Read the model definition and answer for the solid it produces. Units are mm, in the model's axes. Coordinates: 2 decimals unless noted, no trailing zeros. Order: outer loops, then holes, each group sorted by start corner. A loop starts at its lowest first (then second) coordinate and runs counter-clockwise, first axis right, second up. Notation, with made-up numbers: (-23, 33) - (17, 33) arc R12 cw to (17, 37) - close; hole circle Ø4 at (83, -3). An arc over 180 degrees is marked (long way). Answer as a JSON object with one key per item and string values. Group by question number.
from build123d import *

# Parameters (mm, degrees)
BOSS_EXTRUDE1_DEPTH = 3
SKETCH2_R           = 1.95
CUT_EXTRUDE1_DEPTH  = 4


with BuildPart() as part:
    # Sketch1 → Boss-Extrude1 (new body)
    with BuildSketch(Plane(origin=(0, 0, 0), x_dir=(1, 0, 0), z_dir=(0, 1, 0))):
        with BuildLine():
            Line((-54, 0), (-2, 0))
            ThreePointArc((-2, 0), (-0.585786438, -0.585786438), (0, -2))
            Line((0, -2), (0, -13))
            ThreePointArc((0, -13), (-0.585786438, -14.414213562), (-2, -15))
            Line((-2, -15), (-54, -15))
            ThreePointArc((-54, -15), (-55.414213562, -14.414213562), (-56, -13))
            Line((-56, -13), (-56, -2))
            ThreePointArc((-56, -2), (-55.414213562, -0.585786438), (-54, 0))
        make_face()
    extrude(amount=BOSS_EXTRUDE1_DEPTH)

    # Sketch2 → Cut-Extrude1 (cut, through all)
    with BuildSketch(Plane(origin=(0, 3, 0), x_dir=(1, 0, 0), z_dir=(0, 1, 0))):
        with Locations((-4, -4)):
            Circle(SKETCH2_R)
        with Locations((-12, -4)):
            Circle(SKETCH2_R)
        with Locations((-76, -4)):
            Circle(SKETCH2_R)
        with Locations((-68, -4)):
            Circle(SKETCH2_R)
        with Locations((-60, -4)):
            Circle(SKETCH2_R)
        with Locations((-52, -4)):
            Circle(SKETCH2_R)
        with Locations((-44, -4)):
            Circle(SKETCH2_R)
        with Locations((-36, -4)):
            Circle(SKETCH2_R)
        with Locations((-28, -4)):
            Circle(SKETCH2_R)
        with Locations((-20, -4)):
            Circle(SKETCH2_R)
    extrude(amount=-CUT_EXTRUDE1_DEPTH, mode=Mode.SUBTRACT)


solid = part.part
1. A cutting plane is placed at B-B on y = 1.7. Write down the section's boundary in (x, z), and give its area (3 significant figures).
2. A cutting plane is placed at C-C on z = 4. State how many separate pieces and enclosed holes the cut face has, and give its area (3 significant figures).
3. Straight lines are drawn through the part: L1, parallel to Z at x = -52, y = 1.5; L2, parallel to Z at x = -29, y = 0.6; L3, parallel to X at y = 1.1, z = 1.5. For each, find the intervals that lie inside material, in ascending order.
4. A cutting plane is placed at D-D on x = -11. Write down the section's boundary in (y, z).
5. For a pull along X with two mould halves and no side action, classify faces 1 (the flat face through (0, 1, 7)), 2 (the cylindrical face through (-26.2, 1.52, 4.75)), 3 (the flat face through (-56, 1, 8)), 4 (the cylindrical face through (-34.2, 1.52, 4.75)) as pulls with the +X half, pulls with the -X half, needs draft (parallel to the pull), parting line crosses it, or undercut.
6. A cutting plane is placed at A-A on x = -52. Write down the section's boundary in (y, z), and give its area (3 significant figures).
Derived:
{
 "1": {"outline": "(-56, 2) arc R2 ccw to (-54, 0) - (-2, 0) arc R2 ccw to (0, 2) - (0, 13) arc R2 ccw to (-2, 15) - (-54, 15) arc R2 ccw to (-56, 13) - close; hole circle Ø3.9 at (-52, 4); hole circle Ø3.9 at (-44, 4); hole circle Ø3.9 at (-36, 4); hole circle Ø3.9 at (-28, 4); hole circle Ø3.9 at (-20, 4); hole circle Ø3.9 at (-12, 4); hole circle Ø3.9 at (-4, 4)", "area": "753 mm2"},
 "2": {"separate pieces": "8", "enclosed holes": "0", "area": "86.1 mm2"},
 "3": {"L1": "z = 0 to 2.05, 5.95 to 15", "L2": "z = 0 to 2.33, 5.67 to 15", "L3": "x = -55.94 to -0.06"},
 "4": {"outline": "(0, 0) - (3, 0) - (3, 2.33) - (0, 2.33) - close; (0, 5.67) - (3, 5.67) - (3, 15) - (0, 15) - close"},
 "5": {"face 1": "pulls with the +X half", "face 2": "undercut", "face 3": "pulls with the -X half", "face 4": "undercut"},
 "6": {"outline": "(0, 0) - (3, 0) - (3, 2.05) - (0, 2.05) - close; (0, 5.95) - (3, 5.95) - (3, 15) - (0, 15) - close", "area": "33.3 mm2"}
}
